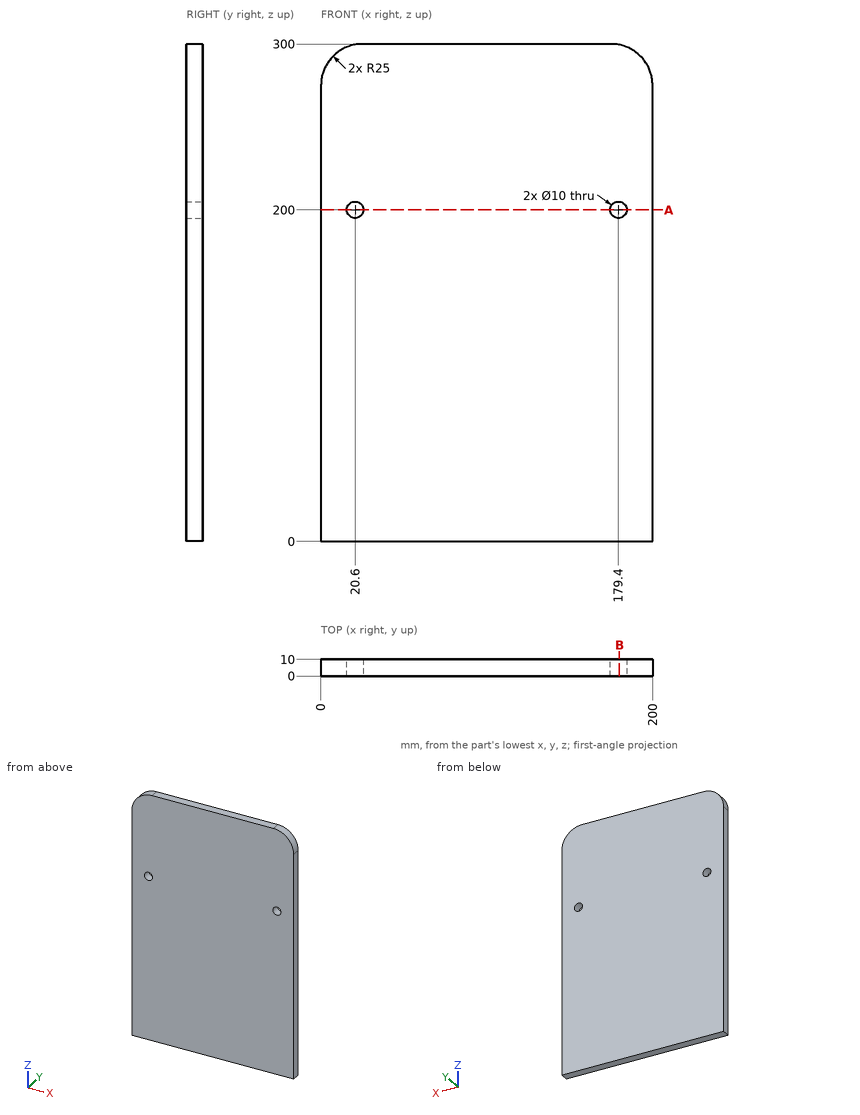
Geometry check sheet. Reference: drawing and pictorial views, mm from the part's lowest x, y, z. Coordinates: 2 decimals unless noted, no trailing zeros. Order: outer loops, then holes, each group sorted by start corner. A loop starts at its lowest first (then second) coordinate and runs counter-clockwise, first axis right, second up. Notation, with made-up numbers: (-20.5, 43) -> (11.5, 43) arc R27 cw to (11.5, 60) -> close; hole circle Ø9 at (69, -38.5). An arc over 180 degrees is marked (long way). Put each result on its own line as item: value. Start each with the question number.
1) Cross-section at B-B (x = 180). Enter the section's corners in (y, z).
2) Cross-section at A-A (z = 200). Enter the section's corners in (x, y), plus the area to 3 significant figures.
3) Go/stop test with a flat-tipped pin: pin 1 (8 mm diameter, centred on x = 179.4, z = 200, fed in from +Y). Record where the tip stops, or that it passes through.
4) Material ranges on L1, parallel to X at y = 5.5, z = 200; L2, parallel to Z at x = 179.4, y = 5.75, recorded low to high.
Geometry check:
1. outline: (0, 0) -> (10, 0) -> (10, 195.04) -> (0, 195.04) -> close; (0, 204.96) -> (10, 204.96) -> (10, 299.49) -> (0, 299.49) -> close
2. outline: (0, 0) -> (15.6, 0) -> (15.6, 10) -> (0, 10) -> close; (25.6, 0) -> (174.4, 0) -> (174.4, 10) -> (25.6, 10) -> close; (184.4, 0) -> (200, 0) -> (200, 10) -> (184.4, 10) -> close
2. area: 1,800 mm^2
3. pin 1: passes through
4. L1: x = 0 to 15.6, 25.6 to 174.4, 184.4 to 200
4. L2: z = 0 to 195, 205 to 299.61
